Geometry check sheet. Reference: the model listing, model coordinates, mm. A direction names the side the tool comes from. Give positions to 0.01 mm unless a question says otherwise; leave off trailing zeros. Loops run counter-clockwise (first coordinate to the right, second up) from the corner with the lowest first, then second, coordinate; pieces in that order, holes last. Notation, with made-up numbers: (-2, 18.5) - (19, 18.5) arc R9 ccw to (19, 29.5) - close; hole circle Ø9 at (10.25, 4.5). An arc over 180 degrees is marked (long way). Use a Markdown table: item, result. Add a question column.
1. Cross-section at B-B on x = 7.75. Enter the section's corners in (y, z).
2. Set-up check for faces 1 (the flat face through (12, 1, 1.5)), 2 (the flat face through (12, -1, -1.5)), 3 (the flat face through (0, -3, 0)): record each of +Z, -Z, +X, -X, +Y, -Y from which the full face is reachable in a straight line by a thin tool's end or side.
3. Cross-section at A-A on y = 11. Enter the section's corners in (x, z).
4. Material ranges on L1, parallel to Y at x = 16, z = -0.15; L2, parallel to Z at x = 1.9, y = 165 (3 decimals); L3, parallel to X at y = 37.5, z = -28, recorded low to high.
5. Depth check by flat-ended pin: P1, Ø2, axis at y = 139.2, z = 87.5, coming from the -X side; P2, Ø6, axis at y = -113.4, z = 87.5, coming from the +X side; P3, Ø7, axis at x = 19.5, y = -18, coming from the +Z side; P4, Ø2.5, axis at x = 14.5, z = 0.5, coming from the +Y side. Enter the tip coordinate at first touch or a pass-through.
6. Cross-section at C-C on z = 42.5. Enter the section's corners in (x, y).
Autodesk Inventor part; units mm, degrees
ref_plane "YZ Plane" through (0, 0, 0) normal (1, 0, 0) x (0, 1, 0)
ref_plane "XZ Plane" through (0, 0, 0) normal (0, 1, 0) x (-1, 0, 0)
ref_plane "XY Plane" through (0, 0, 0) normal (0, 0, 1) x (1, 0, 0)
sketch "Sketch1" plane through (0, 0, 0) normal (1, 0, 0) x (0, 1, 0)
  line L0 (180, 100) -> (-180, 100)
  line L1 (-180, 100) -> (-180, -100)
  line L2 (-180, -100) -> (180, -100)
  line L3 (180, -100) -> (180, 100)
  line L4 (180, 100) -> (-180, -100) construction
  line L5 (-180, 100) -> (180, -100) construction
  point P0 (0, 0)
  dimension "d0" = 360
  dimension "d1" = 200
extrude "Extrusion1" add sketch "Sketch1" along normal blind 3
sketch "Sketch7" plane through (3, 0, 0) normal (1, 0, 0) x (0, 0, -1)
  line L0 (1.5, 50) -> (-1.5, 50)
  line L1 (-1.5, 50) -> (-1.5, -50)
  line L2 (-1.5, -50) -> (1.5, -50)
  line L3 (1.5, -50) -> (1.5, 50)
  line L4 (1.5, 50) -> (-1.5, -50) construction
  line L5 (-1.5, 50) -> (1.5, -50) construction
  point P0 (0, 0)
  dimension "d69" = 3
  dimension "d70" = 100
extrude "Extrusion10" add sketch "Sketch7" along normal blind 24
sketch "Sketch8" plane through (3, -50, 1.5) normal (0, 0, 1) x (1, 0, 0)
  circle A0 centre (13, 75) radius 1.5
  circle A1 centre (13, 50) radius 1.5
  circle A2 centre (13, 25) radius 1.5
  line L0 (0, 100) -> (24, 100)
  line L1 (0, 0) -> (24, 0)
  line L2 (24, 100) -> (24, 0)
  line L3 (0, 230) -> (0, -130)
  point P0 (-3, 50)
  dimension "d73" = 3
  dimension "d74" = 3
  dimension "d75" = 3
  dimension "d76" = 25
  dimension "d77" = 25
  dimension "d78" = 25
  dimension "d87" = 25
  dimension "d88" = 11
  dimension "d89" = 11
  dimension "d90" = 11
extrude "Extrusion11" cut sketch "Sketch8" against normal blind 25 contours A0 | A1 | A2
sketch "Sketch9" plane through (3, 0, 0) normal (1, 0, 0) x (0, 0, -1)
  circle A0 centre (-87.5, 165) radius 1.875
  circle A1 centre (-87.5, 139.2) radius 1.875
  circle A2 centre (-87.5, 113.4) radius 1.875
  line L0 (100, 180) -> (-100, 180)
  line L1 (-100, 180) -> (-100, -180)
  point P0 (0, 0)
  dimension "d91" = 3.75
  dimension "d92" = 3.75
  dimension "d93" = 3.75
  dimension "d96" = 15
  dimension "d97" = 25.8
  dimension "d98" = 25.8
  dimension "d99" = 12.5
extrude "Extrusion12" cut sketch "Sketch9" against normal blind 10
mirror "Mirror2" about plane through (0, 0, 0) normal (0, 1, 0) of "Extrusion12"
sketch "Sketch10" plane through (3, 0, 0) normal (1, 0, 0) x (0, 0, -1)
  line L0 (100, 180) -> (-100, 180)
  line L1 (-100, 180) -> (-97.5, 180)
  line L2 (-97.5, 180) -> (-97.5, -180)
  line L3 (-100, -180) -> (100, -180)
  line L4 (-97.5, -180) -> (-100, -180)
  line L5 (-100, -180) -> (-100, 180)
  point P0 (0, 0)
  dimension "d102" = 2.5
  dimension "d103" = 90
extrude "Extrusion13" cut sketch "Sketch10" against normal blind 10
properties part number "leftside"
Values found:
| question | item | result |
|---|---|---|
| 1 | outline | (-50, -1.5) - (50, -1.5) - (50, 1.5) - (-50, 1.5) - close |
| 2 | face 1 | +Z, +X, +Y, -Y |
| 2 | face 2 | -Z, +X, +Y, -Y |
| 2 | face 3 | +Z, -Z, -X, +Y, -Y |
| 3 | outline | (0, -100) - (3, -100) - (3, -1.5) - (27, -1.5) - (27, 1.5) - (3, 1.5) - (3, 97.5) - (0, 97.5) - close |
| 4 | L1 | y = -50 to -26.5, -23.5 to -1.5, 1.5 to 23.5, 26.5 to 50 |
| 4 | L2 | z = -100 to 85.625, 89.375 to 97.5 |
| 4 | L3 | x = 0 to 3 |
| 5 | P1 | passes through |
| 5 | P2 | stops at x = 3 |
| 5 | P3 | stops at z = 1.5 |
| 5 | P4 | stops at y = 50 |
| 6 | outline | (0, -180) - (3, -180) - (3, 180) - (0, 180) - close |
